Can you work these out from the model? Positions are in its coordinate system, mm. A direction names the side the tool comes from. Round coordinates to 2 decimals unless told otherwise and drop trailing zeros. Loops run counter-clockwise (first coordinate to the right, second up) from the corner with the lowest first, then second, coordinate; pieces in that order, holes last. Notation, with made-up numbers: (13, -2) -> (45, -2) arc R27 ccw to (45, 30) -> close; hole circle Ø8 at (39.5, -35.75). An arc over 180 degrees is marked (long way). Use a Markdown table: item, result.
Autodesk Inventor part; units mm, degrees
ref_plane "YZ Plane" through (0, 0, 0) normal (1, 0, 0) x (0, 1, 0)
ref_plane "XZ Plane" through (0, 0, 0) normal (0, 1, 0) x (-1, 0, 0)
ref_plane "XY Plane" through (0, 0, 0) normal (0, 0, 1) x (1, 0, 0)
sketch "Sketch1" plane through (0, 0, 0) normal (0, 0, 1) x (1, 0, 0)
  circle A0 centre (0, 0) radius 22.5
  circle A1 centre (0, 0) radius 25
  dimension "d2" = 45
  dimension "d3" = 50
extrude "Extrusion1" add sketch "Sketch1" against normal blind 40
sketch "Sketch2" plane through (0, 0, 0) normal (0, 0, 1) x (1, 0, 0)
  circle A0 centre (0, 0) radius 22.5
  circle A1 centre (0, 0) radius 29.5096
extrude "Extrusion2" add sketch "Sketch2" along normal blind 7
sketch "Sketch3" plane through (0, 0, 7) normal (0, 0, 1) x (1, 0, 0)
  line L0 (22.6433, -19.1315) -> (13.1623, -147.983)
  arc A0 (-13.1623, -147.983) -> (13.1623, -147.983) centre (0, -147.0145) ccw
  circle A1 centre (0, 0) radius 29.5096
  line L1 (0, -29.5096) -> (0, -45.4675)
  line L2 (-22.6433, -19.1315) -> (-13.1623, -147.983)
  line L3 (-22.6433, -19.1315) -> (0, -26.0827)
  line L4 (0, -26.0827) -> (22.6433, -19.1315)
  circle A2 centre (0, -147.0145) radius 7.452
extrude "Extrusion3" add sketch "Sketch3" against normal blind 7 contours L0 A0 L2 L3 A1 L4 | A1 L3 L4 picked at (-13.395, -22.9465)
properties part number "Manivelle"
1. I want a section at B-B (y = 0). Please give me the cut outline in (x, z).
Answer sheet:
| item | result |
|---|---|
| outline | (-29.51, 0) -> (-25, 0) -> (-25, -40) -> (-22.5, -40) -> (-22.5, 7) -> (-29.51, 7) -> close; (22.5, -40) -> (25, -40) -> (25, 0) -> (29.51, 0) -> (29.51, 7) -> (22.5, 7) -> close |
2. Which directions (+Z, -Z, +X, -X, +Y, -Y) give clear straight access to the entire face, cutting with the end or side of a thin tool? Please do faces 1 (the flat face through (17.97, -82.66, 3.55)), 2 (the cylindrical face through (23.846, 7.509, -19.72)).
Answer sheet:
| item | result |
|---|---|
| face 1 | +Z, -Z, +X, -Y |
| face 2 | -Z |
3. I want a section at A-A (x = 0). Please give me the cut outline in (y, z).
Answer sheet:
| item | result |
|---|---|
| outline | (-160.21, 0) -> (-154.47, 0) -> (-154.47, 7) -> (-160.21, 7) -> close; (-139.56, 0) -> (-25, 0) -> (-25, -40) -> (-22.5, -40) -> (-22.5, 7) -> (-139.56, 7) -> close; (22.5, -40) -> (25, -40) -> (25, 0) -> (29.51, 0) -> (29.51, 7) -> (22.5, 7) -> close |
4. If we mould it in two halves opening along X, with no side actions, what happens to faces 3 (the cylindrical face through (10.382, -19.961, -16.171)), 4 (the cylindrical face through (-0.28, -160.21, 3.55)), 5 (the flat face through (0, -64, 7))? For each: +X half, -X half, draft (parallel to the pull), parting line (faces both ways), or undercut.
Answer sheet:
| item | result |
|---|---|
| face 3 | undercut |
| face 4 | parting line |
| face 5 | draft |
5. I want a section at D-D (z = -21.5). Please give me the cut outline in (x, y).
Answer sheet:
| item | result |
|---|---|
| outline | circle Ø50 at (0, 0); hole circle Ø45 at (0, 0) |
6. I need wall thicknesses on line 1 (Y direction, x = 0, z = -24); line 2 (Z direction, x = 7, y = -133.5); line 3 (X direction, y = 20, z = -4.5). Which ranges of each line are inside material? Lowest first, please.
Answer sheet:
| item | result |
|---|---|
| line 1 | y = -25 to -22.5, 22.5 to 25 |
| line 2 | z = 0 to 7 |
| line 3 | x = -15 to -10.31, 10.31 to 15 |
7. I want a section at C-C (x = 11). Please give me the cut outline in (y, z), plus the area to 3 significant figures.
Answer sheet:
| item | result |
|---|---|
| outline | (-154.31, 0) -> (-22.45, 0) -> (-22.45, -40) -> (-19.63, -40) -> (-19.63, 7) -> (-154.31, 7) -> close; (19.63, -40) -> (22.45, -40) -> (22.45, 0) -> (27.38, 0) -> (27.38, 7) -> (19.63, 7) -> close |
| area | 1,220 mm² |
8. Will these pins go through, and if not, where does the flat tip stop? pin 1 Ø10 at (x, z) = (5.5, -26.5) entering from -Y (3 decimals); pin 2 Ø10 at (x, y) = (-13.5, 10) entering from -Z; pin 3 Ø2 at (x, y) = (14, -83.5) entering from -Z; pin 4 Ø8 at (y, z) = (9.5, -18) entering from +X.
Answer sheet:
| item | result |
|---|---|
| pin 1 | stops at y = -24.995 |
| pin 2 | passes through |
| pin 3 | stops at z = 0 |
| pin 4 | stops at x = 24.39 |
